The model under review builds one solid part; all positions refer to its coordinate system, in mm. Face numbers are marked on the shaded views. A direction names the side the tool comes from. Round coordinates to 2 decimals unless told otherwise and drop trailing zeros. Write each loop counter-clockwise with the first axis right and the second up, starting at its lowest first coordinate (ties: lowest second). Pieces come first, ordered by that corner, then holes. Notation, with made-up numbers: (-23.5, 1.5) - (-2.5, 1.5) arc R30 ccw to (-2.5, 37.5) - close; hole circle Ø2 at (4.5, -20). An arc over 180 degrees is marked (long way). Return JSON: item names as keys, results as strings.
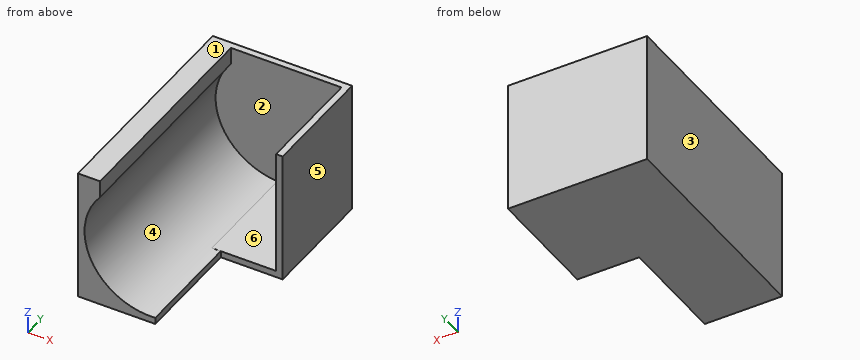
from build123d import *

# Parameters (mm, degrees)
SKETCH1_W           = 60
SKETCH1_H           = 100
BOSS_EXTRUDE1_DEPTH = 3
SKETCH2_W           = 3
SKETCH2_H           = 50
BOSS_EXTRUDE2_DEPTH = 60
SKETCH3_W           = 3
SKETCH3_H           = 50
BOSS_EXTRUDE3_DEPTH = 57
SKETCH4_W           = 63
SKETCH4_H           = 60
BOSS_EXTRUDE4_DEPTH = 3
BOSS_EXTRUDE6_REACH = 123.939


with BuildPart() as part:
    # Sketch1 → Boss-Extrude1 (new body)
    with BuildSketch(Plane(origin=(0, 0, 0), x_dir=(0, 0, -1), z_dir=(1, 0, 0))):
        Rectangle(SKETCH1_W, SKETCH1_H)
    extrude(amount=BOSS_EXTRUDE1_DEPTH)

    # Sketch2 → Boss-Extrude2 (add)
    with BuildSketch(Plane(origin=(3, 0, 0), x_dir=(0, 0, -1), z_dir=(1, 0, 0))):
        with Locations((28.5, 25)):
            Rectangle(SKETCH2_W, SKETCH2_H)
    extrude(amount=BOSS_EXTRUDE2_DEPTH)

    # Sketch3 → Boss-Extrude3 (add)
    with BuildSketch(Plane.XY.offset(-27)):
        with Locations((61.5, 25)):
            Rectangle(SKETCH3_W, SKETCH3_H)
    extrude(amount=BOSS_EXTRUDE3_DEPTH)

    # Sketch4 → Boss-Extrude4 (add)
    with BuildSketch(Plane(origin=(0, 50, 0), x_dir=(1, 0, 0), z_dir=(0, 1, 0))):
        with Locations((31.5, 0)):
            Rectangle(SKETCH4_W, SKETCH4_H)
    extrude(amount=BOSS_EXTRUDE4_DEPTH)

    # Boss-Extrude6: up to this face of the body (flat: up to its plane)
    boss_extrude6_end = Plane(part.part.faces().sort_by_distance((1.5, -50, 0))[0])
    # Sketch7 → Boss-Extrude6 (add, up to the picked face)
    with BuildSketch(Plane.XZ.offset(-50), mode=Mode.PRIVATE) as boss_extrude6_sk1:
        with BuildLine():
            Line((0, -30), (35, -30))
            Line((35, -30), (35, -27))
            ThreePointArc((35, -27), (6.255324942, -10.658001188), (10, 22.194619378))
            Line((10, 22.194619378), (10, 30))
            Line((10, 30), (0, 30))
            Line((0, 30), (0, -30))
        make_face()
    boss_extrude6_tool1 = split(extrude(boss_extrude6_sk1.sketch, amount=BOSS_EXTRUDE6_REACH, mode=Mode.PRIVATE), bisect_by=boss_extrude6_end, keep=Keep.BOTH, mode=Mode.PRIVATE)
    add(boss_extrude6_tool1.solids().sort_by(Axis((17.5, 50, -29.305378), (0, -1, 0)))[0])


solid = part.part
(1) Wall thickness on line 1 (Y direction, x = 20.5, z = -14); line 2 (X direction, y = 19, z = 19); line 3 (X direction, y = 18.5, z = -17.5): over which ranges is each line inside the solid? List them lowest first.
Filled in:
{"line 1": "y = 50 to 53", "line 2": "x = 0 to 7.67, 60 to 63", "line 3": "x = 0 to 11.03, 60 to 63"}
(2) Add section D-D (y = -6.5). Write out the cut boundary in (x, z), plus the area to 3 significant figures.
Filled in:
{"outline": "(0, -30) - (35, -30) - (35, -27) arc R30 cw to (10, 22.19) - (10, 30) - (0, 30) - close", "area": "564 mm2"}
(3) Add section A-A (y = 38). Write out the cut boundary in (x, z), plus the area to 3 significant figures.
Filled in:
{"outline": "(0, -30) - (63, -30) - (63, 30) - (60, 30) - (60, -27) - (31, -27) arc R30 cw to (10, 22.19) - (10, 30) - (0, 30) - close", "area": "819 mm2"}
(4) Clearance check with flat-ended pins moving along their axes: pin 1 Ø25 at (y, z) = (31, -7) entering from -X; pin 2 Ø2.5 at (y, z) = (-35, -28.5) entering from +X; pin 3 Ø3 at (y, z) = (-21.5, -9.5) entering from +X; pin 4 Ø14 at (x, z) = (49.5, 3) entering from -Y. State where each tip first meets the part, or that it passes through.
Filled in:
{"pin 1": "stops at x = 0", "pin 2": "stops at x = 35", "pin 3": "stops at x = 6.43", "pin 4": "stops at y = 50"}
(5) Add section B-B (z = 26.5). Write out the cut boundary in (x, y), plus the area to 3 significant figures.
Filled in:
{"outline": "(0, -50) - (10, -50) - (10, 50) - (60, 50) - (60, 0) - (63, 0) - (63, 53) - (0, 53) - close", "area": "1,340 mm2"}
(6) Mouldability with a two-part tool opening along X and no side actions: class the marked faces 1, 2 and 3 as released by +X, released by -X, zero draft, split by the parting line, or undercut.
Filled in:
{"face 1": "zero draft", "face 2": "undercut", "face 3": "released by -X"}
(7) For the marked faces 4, 5 and 6, list the 3-axis set-ups (+Z, -Z, +X, -X, +Y, -Y) from which the entire face can be reached by the end or side of a thin tool; tool diameter is ignored.
Filled in:
{"face 4": "-Y", "face 5": "+Z, -Z, +X, +Y, -Y", "face 6": "+Z, -Y"}
(8) Add section C-C (x = 55). Write out the cut boundary in (y, z), plus the area to 3 significant figures.
Filled in:
{"outline": "(0, -30) - (53, -30) - (53, 30) - (50, 30) - (50, -27) - (0, -27) - close", "area": "330 mm2"}
